Autodesk Inventor part; units mm, degrees
ref_plane "YZ Plane" through (0, 0, 0) normal (1, 0, 0) x (0, 1, 0)
ref_plane "XZ Plane" through (0, 0, 0) normal (0, 1, 0) x (-1, 0, 0)
ref_plane "XY Plane" through (0, 0, 0) normal (0, 0, 1) x (1, 0, 0)
sketch "Sketch1" plane through (0, 0, 0) normal (0, 1, 0) x (-1, 0, 0)
  line L0 (-35, 46.5) -> (35, 46.5)
  line L1 (35, 46.5) -> (35, -46.5)
  line L2 (35, -46.5) -> (-35, -46.5)
  line L3 (-35, -46.5) -> (-35, 46.5)
  line L4 (-35, 46.5) -> (35, -46.5) construction
  line L5 (35, 46.5) -> (-35, -46.5) construction
  line L6 (-22.5, 37.5) -> (22.5, 37.5)
  line L7 (22.5, 37.5) -> (22.5, -37.5)
  line L8 (22.5, -37.5) -> (-22.5, -37.5)
  line L9 (-22.5, -37.5) -> (-22.5, 37.5)
  line L10 (-22.5, 37.5) -> (22.5, -37.5) construction
  line L11 (22.5, 37.5) -> (-22.5, -37.5) construction
  point P0 (0, 0)
  dimension "d0" = 70
  dimension "d1" = 93
  dimension "d2" = 45
  dimension "d3" = 75
extrude "Extrusion1" add sketch "Sketch1" against normal blind 1.6 contours L0 L1 L2 L3 | L6 L7 L8 L9
extrude "Extrusion2" add sketch "Sketch1" along normal blind 9.7 contours L6 L7 L8 L9
sketch "Sketch2" plane through (0, 9.7, 0) normal (0, 1, 0) x (1, 0, 0)
  line L0 (20, -35) -> (-20, -35)
  line L1 (-20, -35) -> (-20, 35)
  line L2 (-20, 35) -> (20, 35)
  line L3 (20, 35) -> (20, -35)
  line L4 (20, -35) -> (-20, 35) construction
  line L5 (-20, -35) -> (20, 35) construction
  point P0 (0, 0)
  dimension "d8" = 40
  dimension "d9" = 70
extrude "Extrusion3" cut sketch "Sketch2" against normal blind 1
properties part number "LCD12864"
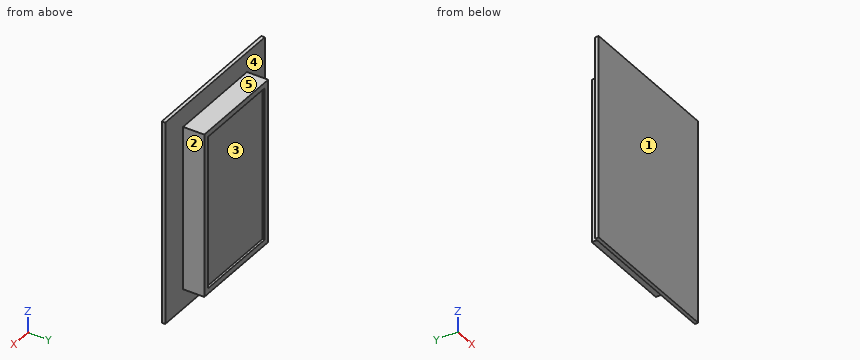
Read the model definition and answer for the solid it produces. Units are mm, in the model's axes. Face numbers are marked on the shaded views. A direction names the side the tool comes from. Round coordinates to 2 decimals unless told otherwise and drop trailing zeros. Loops run counter-clockwise (first coordinate to the right, second up) from the corner with the lowest first, then second, coordinate; pieces in that order, holes last. Notation, with made-up numbers: (42.5, -1.5) - (97.5, -1.5) arc R25 ccw to (97.5, 19.5) - close; hole circle Ø3 at (-22, 77). An arc over 180 degrees is marked (long way). One line per question, with ' | ' between items. Start each with the question number.
Q1. For a pull along Z with two mould halves and no side action, classify the marked faces 3, 4 and 5 as +Z half, -Z half, draft (parallel to the pull), parting line (faces both ways), or undercut.
Q2. Section D-D on x = -30 is taken. Give the vertices of the cut face in (y, z), plus the area to 3 significant figures.
Q3. Flat-ended cylindrical pins translate along their axes: pin 1 (6 mm diameter, centred on x = -27.5, z = -31.5, fed in from +Y); pin 2 (4 mm diameter, centred on x = -17, y = 3.5, fed in from -Z); pin 3 (1 mm diameter, centred on x = -15, z = 19.5, fed in from +Y). Find the tip coordinate at first contact, or state that the pin passes through.
Q4. Find the intervals of material crossed by L1, parallel to X at y = 9, z = -6.5; L2, parallel to Z at x = -19, y = 0.5; L3, parallel to Y at x = -2, z = 27.5, in increasing order.
Q5. Section A-A on x = -3 is taken. Give the vertices of the cut face in (y, z).
Q6. Section C-C on y = 7.25 is taken. Give the vertices of the cut face in (x, z), plus the area to 4 significant figures.
Q7. Section B-B on z = -6.5 is taken. Give the vertices of the cut face in (x, y), plus the area to 4 significant figures.
Q8. For the marked faces 1 and 2, determine the directions among +Z, -Z, +X, -X, +Y, -Y from which every point of the face is accessible in a straight line to the end or side of a thin tool.
Established:
1) face 3: undercut | face 4: draft | face 5: +Z half
2) outline: (-1.6, -46.5) - (0, -46.5) - (0, 46.5) - (-1.6, 46.5) - close | area: 149 mm²
3) pin 1: y = 0 | pin 2: z = -37.5 | pin 3: y = 8.7
4) L1: -22.5 to -20, 20 to 22.5 | L2: -37.5 to 37.5 | L3: -1.6 to 8.7
5) outline: (-1.6, -46.5) - (0, -46.5) - (0, -37.5) - (9.7, -37.5) - (9.7, -35) - (8.7, -35) - (8.7, 35) - (9.7, 35) - (9.7, 37.5) - (0, 37.5) - (0, 46.5) - (-1.6, 46.5) - close
6) outline: (-22.5, -37.5) - (22.5, -37.5) - (22.5, 37.5) - (-22.5, 37.5) - close | area: 3,375 mm²
7) outline: (-35, -1.6) - (35, -1.6) - (35, 0) - (22.5, 0) - (22.5, 9.7) - (20, 9.7) - (20, 8.7) - (-20, 8.7) - (-20, 9.7) - (-22.5, 9.7) - (-22.5, 0) - (-35, 0) - close | area: 508.5 mm²
8) face 1: +Z, -Z, +X, -X, -Y | face 2: +Z, -Z, +X, +Y
